```python
from build123d import *

# Parameters (mm, degrees)
F3_W     = 25.4
F3_H     = 7.62
F4_DEPTH = 25.4


with BuildPart() as f1:
    # F0 (on Front) → F1 (revolve)
    with BuildSketch(Plane.XZ):
        Polygon((-101.6, 7.9375), (-101.6, 0), (101.6, 0), (101.6, 7.9375), (38.1, 7.9375), (38.1, 12.7), (-38.1, 12.7), (-38.1, 7.9375), align=None)
    revolve(axis=Axis((0, 0, 0), (-1, 0, 0)))

    # F3 (on offset) → F4 (cut)
    with BuildSketch(Plane.XY.offset(12.7)):
        with Locations((0, 12.7)):
            Rectangle(F3_W, F3_H)
        with Locations((0, -12.7)):
            Rectangle(F3_W, F3_H)
    extrude(amount=-F4_DEPTH, mode=Mode.SUBTRACT)


solid = f1.part
```
Read the model definition and answer for the solid it produces. Units are mm, in the model's axes. A direction names the side the tool comes from. Coordinates: 2 decimals unless noted, no trailing zeros. Order: outer loops, then holes, each group sorted by start corner. A loop starts at its lowest first (then second) coordinate and runs counter-clockwise, first axis right, second up. Notation, with made-up numbers: (-27.5, -9) - (-11.5, -9) arc R11 ccw to (-11.5, 5) - close; hole circle Ø8 at (37.5, 15.25). An arc over 180 degrees is marked (long way). Answer as a JSON object with one key per item and string values. Group by question number.
Item 1: Section C-C (x = 2) is taken. Give the vertices of the cut face in (y, z).
Item 2: Flat-ended cylindrical pins translate along their axes: P1, Ø10, axis at x = 69, z = 0.5, coming from the -Y side; P2, Ø9, axis at x = 5, z = 3.5, coming from the -Y side; P3, Ø5, axis at x = 29, z = 7, coming from the -Y side. Find the tip coordinate at first contact, or state that the pin passes through.
Item 3: The mould has two halves that part along X. Classify faces 4 (the face through (-12.7, 10, 0)), 5 (the face through (-70.29, -7.75, -1.72)), 6 (the face through (-101.6, 0, 0)): +X half, -X half, draft (parallel to the pull), parting line (faces both ways), or undercut.
Item 4: Section D-D (x = -66.5) is taken. Give the vertices of the cut face in (y, z) (1 decimal), plus the area to 3 significant figures.
Item 5: Consider probe 1 along X at (y, z) = (11.25, -1); probe 2 along X at (y, z) = (6.5, -8.5); probe 3 along Y at (x, z) = (5.5, 0.5). Determine where each line is inside the solid, lowest interval first. Write a range as from..to.
Item 6: Section B-B (z = 0) is taken. Give the vertices of the cut face in (x, y).
Item 7: Section A-A (y = 0) is taken. Give the vertices of the cut face in (x, z).
Item 8: A tool of negligible diameter and unlimited length cuts with its end or side. For faces 1 (the face through (-38.1, -8.3, -0.2)), 2 (the face through (-12.7, -10, 0)), 3 (the face through (69.41, -7.75, -1.72)), from which of +Z, -Z, +X, -X, +Y, -Y can it reach the whole face along a straight path? Write none if from no direction.
Results are:
{
 "1": {"outline": "(-8.89, -9.07) arc R12.7 ccw to (8.89, -9.07) - (8.89, 9.07) arc R12.7 ccw to (-8.89, 9.07) - close"},
 "2": {"P1": "stops at y = -7.94", "P2": "stops at y = -8.89", "P3": "stops at y = -11.88"},
 "3": {"face 4": "undercut", "face 5": "draft", "face 6": "-X half"},
 "4": {"outline": "circle Ø15.9 at (0, 0)", "area": "198 mm^2"},
 "5": {"probe 1": "x = -38.1..-12.7, 12.7..38.1", "probe 2": "x = -38.1..38.1", "probe 3": "y = -8.89..8.89"},
 "6": {"outline": "(-101.6, -7.94) - (-38.1, -7.94) - (-38.1, -12.7) - (-12.7, -12.7) - (-12.7, -8.89) - (12.7, -8.89) - (12.7, -12.7) - (38.1, -12.7) - (38.1, -7.94) - (101.6, -7.94) - (101.6, 7.94) - (38.1, 7.94) - (38.1, 12.7) - (12.7, 12.7) - (12.7, 8.89) - (-12.7, 8.89) - (-12.7, 12.7) - (-38.1, 12.7) - (-38.1, 7.94) - (-101.6, 7.94) - close"},
 "7": {"outline": "(-101.6, -7.94) - (-38.1, -7.94) - (-38.1, -12.7) - (38.1, -12.7) - (38.1, -7.94) - (101.6, -7.94) - (101.6, 7.94) - (38.1, 7.94) - (38.1, 12.7) - (-38.1, 12.7) - (-38.1, 7.94) - (-101.6, 7.94) - close"},
 "8": {"face 1": "-X", "face 2": "+Z, -Z, -Y", "face 3": "+X"}
}
